Source: CAD feature listing. Evaluate the final solid. Frame: model axes, mm. Face numbers are marked on the shaded views. A direction names the side the tool comes from. Round coordinates to 2 decimals unless told otherwise and drop trailing zeros. Loops run counter-clockwise (first coordinate to the right, second up) from the corner with the lowest first, then second, coordinate; pieces in that order, holes last.
Item 1: Section query C-C on y = 0. Return loops of the section in (x, z).
Item 2: Access query for the marked faces 4 and 5. Directions: +Z, -Z, +X, -X, +Y, -Y. A direction counts if a zero-diameter tool reaches every point of the face in a straight line with its end or side. Return the directions, or none.
Item 3: Ray query, L1, parallel to Y at x = 0, z = 4.6; L2, parallel to Y at x = 0, z = 1.8; L3, parallel to X at y = 8, z = 5.1. Return the intervals inside material, ascending.
Item 4: Pull-direction query (X, two-part tool) for the marked faces 1, 2 and 3; classes: released by +X, released by -X, zero draft, split by the parting line, or undercut.
Item 5: First-contact query: P1, Ø2, axis at x = -9.5, z = 5, coming from the -Y side; P2, Ø1, axis at x = -2, z = 1.5, coming from the +Y side; P3, Ø3.5, axis at x = 8, y = 0, coming from the +Z side. Flat tips, straight axial feed; report the tip coordinate or a pass-through.
Item 6: Section query B-B on z = 0.95. Give the number of separate pieces and of enclosed holes in the cut face, then the cut area to 3 significant figures.
Item 7: Section query A-A on x = 0. Return loops of the section in (y, z).
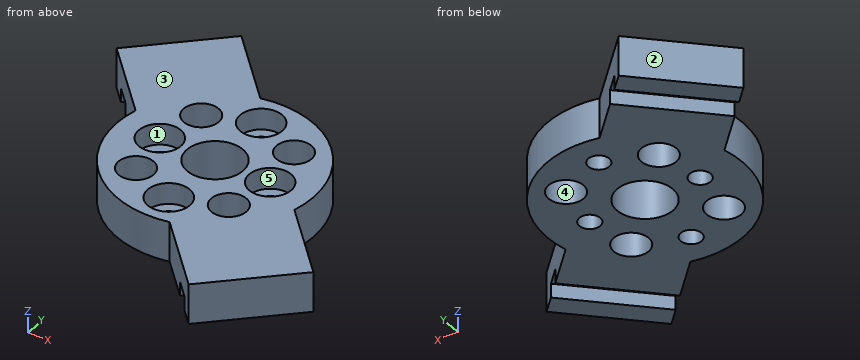
```python
from build123d import *

# Parameters (mm, degrees)
F0_R     = 14
F0_R_2   = 2.5
F0_R_3   = 1.5
F0_R_4   = 4
F1_DEPTH = 5.7
F2_R     = 3
F2_R_2   = 1.5
F3_DEPTH = 3
F5_DEPTH = 5.7
F7_DEPTH = 2


with BuildPart() as f1:
    # F0 (on Top) → F1 (new body)
    with BuildSketch(Plane.XY):
        Circle(F0_R)
        with Locations((-6.707044, -6.727968)):
            Circle(F0_R_2, mode=Mode.SUBTRACT)
        with Locations((0, -9.5)):
            Circle(F0_R_3, mode=Mode.SUBTRACT)
        with Locations((6.727968, -6.707044)):
            Circle(F0_R_2, mode=Mode.SUBTRACT)
        with Locations((-8, 0)):
            Circle(F0_R_3, mode=Mode.SUBTRACT)
        with Locations((-6.727968, 6.707044)):
            Circle(F0_R_2, mode=Mode.SUBTRACT)
        Circle(F0_R_4, mode=Mode.SUBTRACT)
        with Locations((6.707044, 6.727968)):
            Circle(F0_R_2, mode=Mode.SUBTRACT)
        with Locations((8, 0)):
            Circle(F0_R_3, mode=Mode.SUBTRACT)
        with Locations((0, 9.5)):
            Circle(F0_R_3, mode=Mode.SUBTRACT)
    extrude(amount=F1_DEPTH)

    # F2 (on face) → F3 (cut)
    with BuildSketch(Plane.XY.offset(5.7)):
        with Locations((0, 9.5)):
            Circle(F2_R)
        with Locations((0, 9.5)):
            Circle(F2_R_2, mode=Mode.SUBTRACT)
        with Locations((-8, 0)):
            Circle(F2_R)
        with Locations((-8, 0)):
            Circle(F2_R_2, mode=Mode.SUBTRACT)
        with Locations((0, -9.5)):
            Circle(F2_R)
        with Locations((0, -9.5)):
            Circle(F2_R_2, mode=Mode.SUBTRACT)
        with Locations((8, 0)):
            Circle(F2_R)
        with Locations((8, 0)):
            Circle(F2_R_2, mode=Mode.SUBTRACT)
    extrude(amount=-F3_DEPTH, mode=Mode.SUBTRACT)

    # F4 (on face) → F5 (join)
    with BuildSketch(Plane.XY.offset(5.7)):
        with BuildLine():
            Line((-22.98097, 12.374369), (-13.662428, 3.055826))
            ThreePointArc((-13.662428, 3.055826), (-9.899495, 9.899495), (-3.055826, 13.662428))
            Line((-3.055826, 13.662428), (-12.374369, 22.98097))
            Line((-12.374369, 22.98097), (-22.98097, 12.374369))
        make_face()
        with BuildLine():
            Line((12.374369, -22.98097), (22.98097, -12.374369))
            Line((22.98097, -12.374369), (13.662428, -3.055826))
            ThreePointArc((13.662428, -3.055826), (9.899495, -9.899495), (3.055826, -13.662428))
            Line((3.055826, -13.662428), (12.374369, -22.98097))
        make_face()
    extrude(amount=-F5_DEPTH)

    # F6 (on face) → F7 (cut)
    with BuildSketch(Plane(origin=(0, 0, 0), x_dir=(1, 0, 0), z_dir=(0, 0, -1))):
        Polygon((-8.131728, -18.73833), (-18.73833, -8.131728), (-20.85965, -10.253048), (-10.253048, -20.85965), align=None)
        Polygon((20.85965, 10.253048), (10.253048, 20.85965), (8.131728, 18.73833), (18.73833, 8.131728), align=None)
    extrude(amount=-F7_DEPTH, mode=Mode.SUBTRACT)


solid = f1.part
```
Data:
1. outline: (-14, 0) - (-9.5, 0) - (-9.5, 2.7) - (-11, 2.7) - (-11, 5.7) - (-14, 5.7) - close; (-6.5, 0) - (-4, 0) - (-4, 5.7) - (-5, 5.7) - (-5, 2.7) - (-6.5, 2.7) - close; (4, 0) - (6.5, 0) - (6.5, 2.7) - (5, 2.7) - (5, 5.7) - (4, 5.7) - close; (9.5, 0) - (14, 0) - (14, 5.7) - (11, 5.7) - (11, 2.7) - (9.5, 2.7) - close
2. face 4: +Z, -Z
2. face 5: +Z
3. L1: y = -14 to -12.5, -6.5 to -4, 4 to 6.5, 12.5 to 14
3. L2: y = -14 to -11, -8 to -4, 4 to 8, 11 to 14
3. L3: x = -18.61 to -8.87, -4.59 to -2.6, 2.6 to 4.55, 8.86 to 11.49
4. face 1: undercut
4. face 2: released by -X
4. face 3: zero draft
5. P1: stops at y = -11.12
5. P2: stops at y = 13.92
5. P3: stops at z = 2.7
6. separate pieces: 3
6. enclosed holes: 9
6. area: 720 mm2
7. outline: (-14, 0) - (-11, 0) - (-11, 2.7) - (-12.5, 2.7) - (-12.5, 5.7) - (-14, 5.7) - close; (-8, 0) - (-4, 0) - (-4, 5.7) - (-6.5, 5.7) - (-6.5, 2.7) - (-8, 2.7) - close; (4, 0) - (8, 0) - (8, 2.7) - (6.5, 2.7) - (6.5, 5.7) - (4, 5.7) - close; (11, 0) - (14, 0) - (14, 5.7) - (12.5, 5.7) - (12.5, 2.7) - (11, 2.7) - close
